Geometry: see drawing. Coordinates: mm, zero at the bounding-box minimum. A direction names the side the tool comes from. Coordinates: 2 decimals unless noted, no trailing zeros. Write each loop counter-clockwise with the first axis right and the second up, starting at its lowest first coordinate (ties: lowest second). Pieces come first, ordered by that corner, then holes.
1) Line query: L1, parallel to X at y = 3.5, z = 5.5; L2, parallel to Y at x = 72, z = 6.75. Output: solid intervals per line, ascending.
2) Section query B-B (z = 19). Output: boundary loops of the cut face in (x, y).
3) Section query C-C (x = 50). Output: boundary loops of the cut face in (y, z).
4) Section query A-A (y = 29.5). Output: boundary loops of the cut face in (x, z).
5) Pin query (flat end, axial travel): pin 1 Ø6 at (x, z) = (45.5, 7) entering from +Y. Return the tip coordinate at first contact, or that it passes through.
6) Set-up query: the marked faces 1 and 2. Return all of +Z, -Z, +X, -X, +Y, -Y with unobstructed straight access to the full face (end or side cutting, diameter ignored); none if empty.
7) Draft query along X for the marked faces 3, 4 and 5. Return one class per face: pulls with the +X half, pulls with the -X half, needs draft (parallel to the pull), parting line crosses it, or undercut.
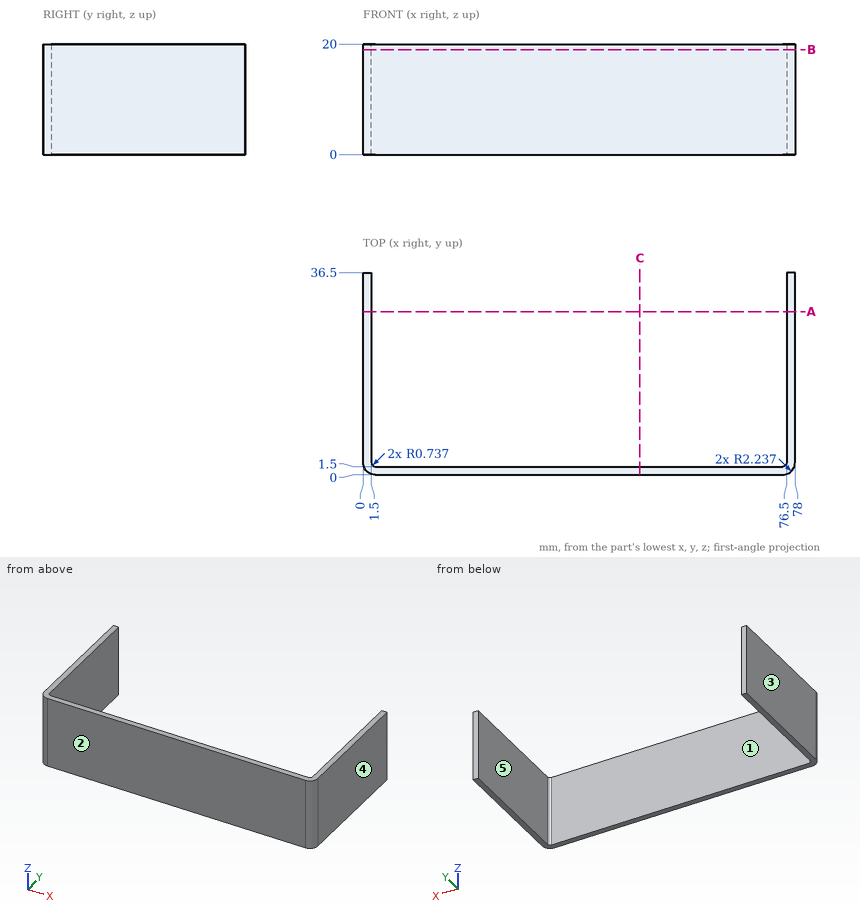
Answer:
1. L1: x = 0 to 1.5, 76.5 to 78
1. L2: y = 0 to 1.5
2. outline: (0, 2.24) arc R2.24 ccw to (2.24, 0) - (75.76, 0) arc R2.24 ccw to (78, 2.24) - (78, 36.5) - (76.5, 36.5) - (76.5, 2.24) arc R0.74 cw to (75.76, 1.5) - (2.24, 1.5) arc R0.74 cw to (1.5, 2.24) - (1.5, 36.5) - (0, 36.5) - close
3. outline: (0, 0) - (1.5, 0) - (1.5, 20) - (0, 20) - close
4. outline: (0, 0) - (1.5, 0) - (1.5, 20) - (0, 20) - close; (76.5, 0) - (78, 0) - (78, 20) - (76.5, 20) - close
5. pin 1: stops at y = 1.5
6. face 1: +Z, -Z, +Y
6. face 2: +Z, -Z, +X, -X, -Y
7. face 3: pulls with the -X half
7. face 4: pulls with the +X half
7. face 5: undercut
